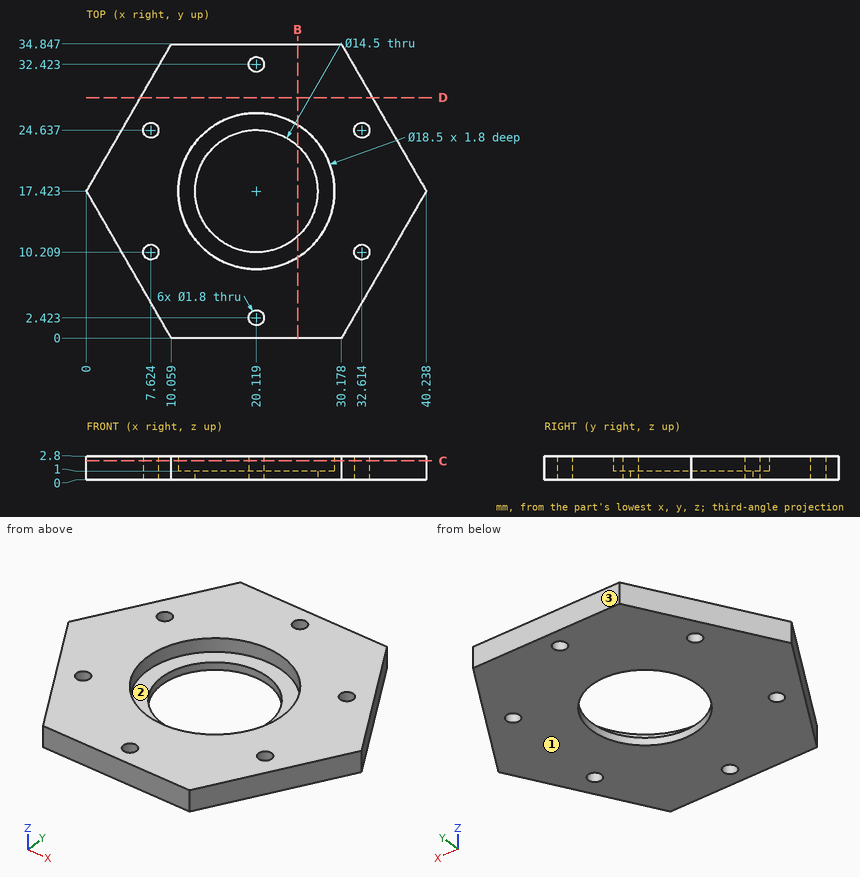
Check sheet for the drawn part. Datum: minimum x, y, z corner. Units: mm. Round coordinates to 2 decimals unless told otherwise and drop trailing zeros. Order: outer loops, then holes, each group sorted by start corner. A loop starts at its lowest first (then second) coordinate and runs counter-clockwise, first axis right, second up. Notation, with made-up numbers: (-32.75, -33) - (-15.75, -33) arc R13 ccw to (-15.75, -27) - close; hole circle Ø5 at (-34, -10.75). An arc over 180 degrees is marked (long way). Use a Markdown table: item, result. Add a question column.
(1) Material ranges on line 1 along Z through (x, y) = (19.5, 9); line 2 along Y through (x, z) = (32.5, 0.7) (1 decimal); line 3 along X through (y, z) = (33, 0.35) (1 decimal), recorded low to high. Write a range as [from, to].
(2) Sectioned sample at D-D, the plane y = 28.5. Enter the section's corners in (x, z) (1 decimal).
(3) Depth check by flat-ended pin: pin 1 (1.4 mm diameter, centred on x = 32.61, y = 10.21, fed in from -Z); pin 2 (4 mm diameter, centred on x = 14, y = 18, fed in from +Z). Enter the tip coordinate at first touch or a pass-through.
(4) Sectioned sample at B-B, the plane x = 25. Enter the section's corners in (y, z) (1 decimal).
(5) Release check for a two-part mould opening along Y. For the marked faces 1, 2 and 3 record: pulls with the +Y half, pulls with the -Y half, needs draft (parallel to the pull), parting line crosses it, or undercut.
(6) Sectioned sample at C-C, the plane z = 2.25. Enter the section's corners in (x, y).
Answers below:
| question | item | result |
|---|---|---|
| 1 | line 1 | [0, 1] |
| 1 | line 2 | [4, 9.3], [11.1, 23.7], [25.5, 30.8] |
| 1 | line 3 | [9, 19.4], [20.8, 31.2] |
| 2 | outline | (6.4, 0) - (33.8, 0) - (33.8, 2.8) - (6.4, 2.8) - close |
| 3 | pin 1 | through |
| 3 | pin 2 | z = 1 |
| 4 | outline | (0, 0) - (12.1, 0) - (12.1, 1) - (9.6, 1) - (9.6, 2.8) - (0, 2.8) - close; (22.8, 0) - (34.8, 0) - (34.8, 2.8) - (25.3, 2.8) - (25.3, 1) - (22.8, 1) - close |
| 5 | face 1 | needs draft |
| 5 | face 2 | undercut |
| 5 | face 3 | pulls with the +Y half |
| 6 | outline | (0, 17.42) - (10.06, 0) - (30.18, 0) - (40.24, 17.42) - (30.18, 34.85) - (10.06, 34.85) - close; hole circle Ø1.8 at (7.62, 10.21); hole circle Ø1.8 at (7.62, 24.64); hole circle Ø18.5 at (20.12, 17.42); hole circle Ø1.8 at (20.12, 2.42); hole circle Ø1.8 at (20.12, 32.42); hole circle Ø1.8 at (32.61, 10.21); hole circle Ø1.8 at (32.61, 24.64) |
